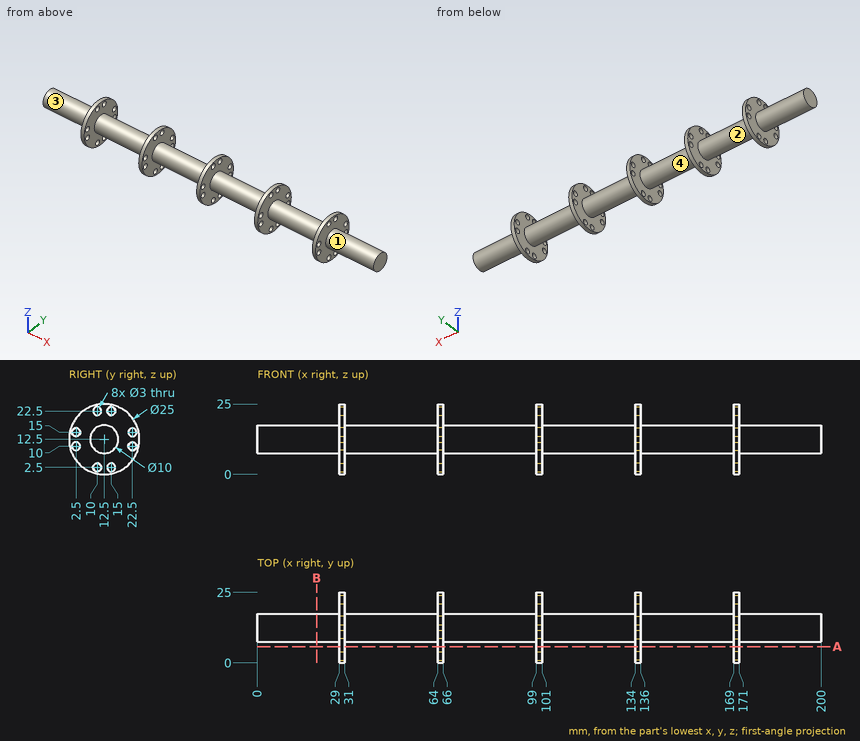
Geometry check sheet. Reference: drawing and pictorial views, mm from the part's lowest x, y, z. A direction names the side the tool comes from. Coordinates: 2 decimals unless noted, no trailing zeros. Write each loop counter-clockwise with the first axis right and the second up, starting at its lowest first coordinate (ties: lowest second). Pieces come first, ordered by that corner, then holes. Notation, with made-up numbers: M 83,76 L 121,76 A20 cw 121,102 Z; hole C -27,69.25 d6. An arc over 180 degrees is marked long. Write item = value, one per line. Start each with the question number.
1. Sectioned sample at A-A (y = 5.75). Record the cut outline in (x, z).
2. Go/stop test with flat-tipped pins: pin 1 (1.8 mm diameter, centred on y = 15, z = 2.5, fed in from +X); pin 2 (2 mm diameter, centred on x = 150.5, z = 15.5, fed in from -Y); pin 3 (10 mm diameter, centred on x = 84.5, z = 16.5, fed in from -Y); pin 4 (3.5 mm diameter, centred on y = 15, z = 2.5, fed in from -X). Record where each tip stops, or that it passes through.
3. Thickness scan on probe 1 along X at (y, z) = (11.5, 23.75); probe 2 along Z at (x, y) = (30.3, 15); probe 3 along Z at (x, y) = (99.7, 2.5). Record the ranges inside material, lowest first.
4. Tool access check on the marked faces 3 and 4. Record the directions out of +Z, -Z, +X, -X, +Y, -Y that give a thin tool (end or side, any length) a straight path to the whole face; none if there is none.
5. Sectioned sample at B-B (x = 21). Record the cut outline in (y, z).
6. Mould release check, pull along X, two halves, no side actions. Record for the marked faces 1 and 2: pulls with the +X half, pulls with the -X half, needs draft (parallel to the pull), parting line crosses it, or undercut.
The answers:
q1.outline = M 29,1.98 L 31,1.98 L 31,23.02 L 29,23.02 Z; M 64,1.98 L 66,1.98 L 66,23.02 L 64,23.02 Z; M 99,1.98 L 101,1.98 L 101,23.02 L 99,23.02 Z; M 134,1.98 L 136,1.98 L 136,23.02 L 134,23.02 Z; M 169,1.98 L 171,1.98 L 171,23.02 L 169,23.02 Z
q2.pin_1 = through
q2.pin_2 = 7.92
q2.pin_3 = 7.5
q2.pin_4 = 29
q3.probe_1 = 29 to 31, 64 to 66, 99 to 101, 134 to 136, 169 to 171
q3.probe_2 = 0.25 to 1, 4 to 21, 24 to 24.75
q3.probe_3 = 5 to 8.5, 11.5 to 13.5, 16.5 to 20
q4.face_3 = -X
q4.face_4 = none
q5.outline = C 12.5,12.5 d10
q6.face_1 = needs draft
q6.face_2 = undercut
